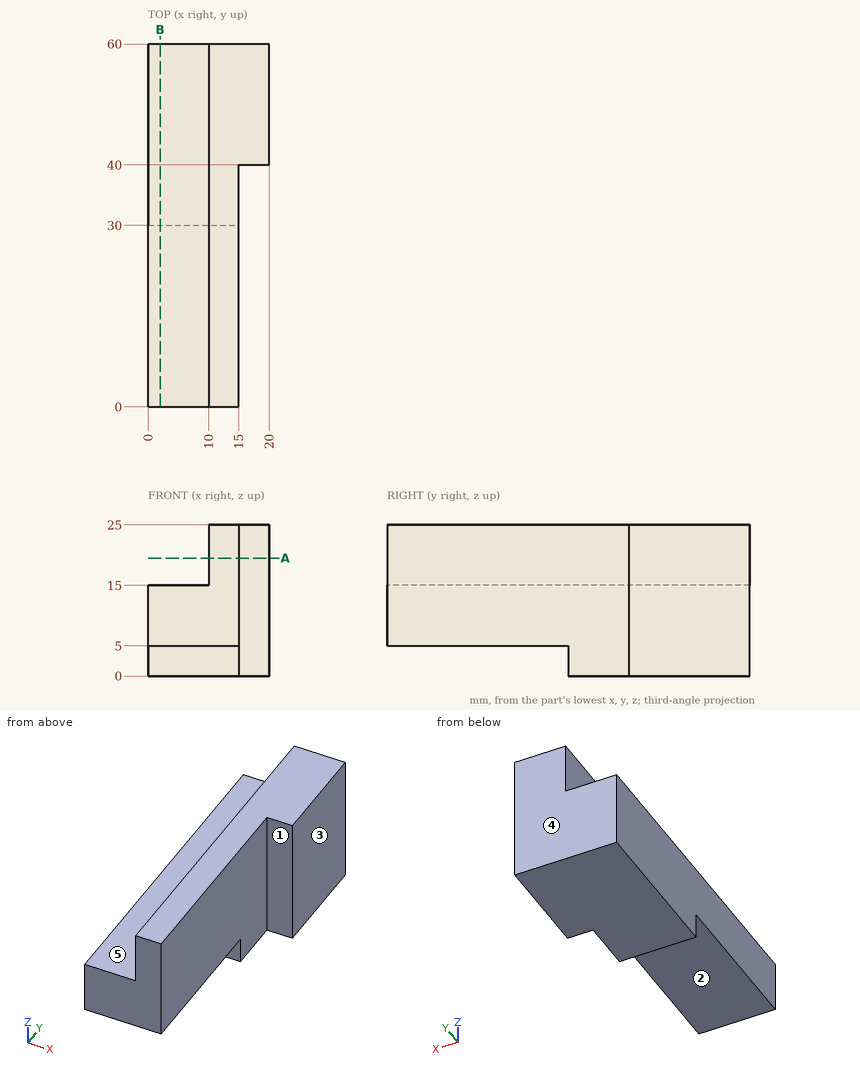
Can you work these out from the drawing? Everything is in mm from the part's minimum corner. A direction names the side the tool comes from. Give positions to 0.01 mm unless a question says otherwise; leave off trailing zeros. Order: outer loops, then holes, each group sorted by start corner. A loop starts at its lowest first (then second) coordinate and runs counter-clockwise, first axis right, second up.
Item 1: If we section it at B-B, the plane x = 2: Write out the boundary of the cut face in (y, z), plus the area to 3 significant figures.
Item 2: I'm going to push flat-ended pins straight in: pin 1 (11 mm diameter, centred on y = 21, z = 18, fed in from -X); pin 2 (4 mm diameter, centred on x = 5, z = 2.5, fed in from -Y); pin 3 (1.5 mm diameter, centred on x = 5, y = 17, fed in from +Z); pin 4 (4.5 mm diameter, centred on x = 10.5, y = 18.5, fed in from -Z). Where does each tip first touch, or does it pass through?
Item 3: I need wall thicknesses on line 1 (Z direction, x = 5.75, y = 33); line 2 (Z direction, x = 3, y = 9); line 3 (X direction, y = 25, z = 22). Which ranges of each line are inside material? Lowest first, please.
Item 4: If we section it at A-A, the plane z = 19.5: Write out the boundary of the cut face in (x, y), plus the area to 3 significant figures.
Item 5: For the marked faces 1, 2, 3, 4 and 5, which set-ups out of +Z, -Z, +X, -X, +Y, -Y let a thin tool reach every point of the face, with its end or its side?
Values:
1. outline: (0, 5) - (30, 5) - (30, 0) - (60, 0) - (60, 15) - (0, 15) - close
1. area: 750 mm2
2. pin 1: stops at x = 0
2. pin 2: stops at y = 30
2. pin 3: stops at z = 15
2. pin 4: stops at z = 5
3. line 1: z = 0 to 15
3. line 2: z = 5 to 15
3. line 3: x = 10 to 15
4. outline: (10, 0) - (15, 0) - (15, 40) - (20, 40) - (20, 60) - (10, 60) - close
4. area: 400 mm2
5. face 1: +Z, -Z, +X, -Y
5. face 2: -Z, +X, -X, -Y
5. face 3: +Z, -Z, +X, +Y, -Y
5. face 4: +Z, -Z, +X, -X, +Y
5. face 5: +Z, -X, +Y, -Y
